Input: part model. Units: mm. Frame: model coordinates. Face numbers are marked on the shaded views. A direction names the side the tool comes from. Round coordinates to 2 decimals unless told otherwise and drop trailing zeros. Loops run counter-clockwise (first coordinate to the right, second up) from the corner with the lowest first, then second, coordinate; pieces in that order, holes last. Notation, with made-up numbers: (-6, 37.25) -> (8, 37.25) arc R22 ccw to (8, 71.25) -> close; hole circle Ø4 at (-12, 42). An arc over 180 degrees is marked (long way). Answer as a JSON object with one key per item and string values.
```python
from build123d import *

# Parameters (mm, degrees)
SKETCH_W        = 54.3
SKETCH_H        = 38
PAD_DEPTH       = 2
SKETCH001_W     = 54.3
SKETCH001_H     = 2
PAD001_DEPTH    = 22
SKETCH002_R     = 2.95
PAD002_DEPTH    = 5
SKETCH003_W     = 40
SKETCH003_H     = 22
PAD003_DEPTH    = 2
SKETCH004_W     = 40
SKETCH004_H     = 22
PAD004_DEPTH    = 2
SKETCH005_W     = 6.85
SKETCH005_H     = 15
PAD005_DEPTH    = 8
SKETCH006_R     = 1.4
POCKET_DEPTH    = 15
FILLET_R        = 3
FILLET001_R     = 2
SKETCH007_W     = 6.85
SKETCH007_H     = 25.8
PAD006_DEPTH    = 20
SKETCH008_R     = 1.4
POCKET001_DEPTH = 15
PAD007_DEPTH    = 2
SKETCH010_R     = 1.4
PAD008_DEPTH    = 2
SKETCH011_R     = 1.4
PAD009_DEPTH    = 2


with BuildPart() as body:
    # Sketch → Pad (new body)
    with BuildSketch(Plane.XY):
        with Locations((27.15, 21)):
            Rectangle(SKETCH_W, SKETCH_H)
    extrude(amount=PAD_DEPTH)

    # Sketch001 → Pad001 (join)
    with BuildSketch(Plane.XY):
        with Locations((27.15, 1)):
            Rectangle(SKETCH001_W, SKETCH001_H)
    extrude(amount=PAD001_DEPTH)

    # Sketch002 → Pad002 (join)
    with BuildSketch(Plane.XZ):
        with Locations((37.25, 12)):
            Circle(SKETCH002_R)
    extrude(amount=PAD002_DEPTH)

    # Sketch003 (on Face2 of Pad002) → Pad003 (join)
    with BuildSketch(Plane(origin=(0, 0, 0), x_dir=(0, -1, 0), z_dir=(-1, 0, 0))):
        with Locations((-20, 11)):
            Rectangle(SKETCH003_W, SKETCH003_H)
    extrude(amount=PAD003_DEPTH)

    # Sketch004 (on Face3 of Pad003) → Pad004 (join)
    with BuildSketch(Plane.YZ.offset(54.3)):
        with Locations((20, 11)):
            Rectangle(SKETCH004_W, SKETCH004_H)
    extrude(amount=PAD004_DEPTH)

    # Sketch005 (on Face5 of Pad004) → Pad005 (join)
    with BuildSketch(Plane.XY.offset(2)):
        with Locations((50.875, 20.3)):
            Rectangle(SKETCH005_W, SKETCH005_H)
    extrude(amount=PAD005_DEPTH)

    # Sketch006 (on Face15 of Pad005) → Pocket (cut)
    with BuildSketch(Plane(origin=(0, 27.8, 0), x_dir=(-1, 0, 0), z_dir=(0, 1, 0))):
        with Locations((-51.3, 7)):
            Circle(SKETCH006_R)
    extrude(amount=-POCKET_DEPTH, mode=Mode.SUBTRACT)

    # Fillet
    fillet_edges = [body.edges().sort_by_distance(p)[0] for p in [
        (47.45, 20.3, 10),
    ]]
    fillet(fillet_edges, radius=FILLET_R)

    # Fillet001
    fillet001_edges = [body.edges().sort_by_distance(p)[0] for p in [
        (52.375, 12.8, 10),
    ]]
    fillet(fillet001_edges, radius=FILLET001_R)

    # Sketch007 (on Face5 of Fillet001) → Pad006 (join)
    with BuildSketch(Plane.XY.offset(2)):
        with Locations((3.425, 14.9)):
            Rectangle(SKETCH007_W, SKETCH007_H)
    extrude(amount=PAD006_DEPTH)

    # Sketch008 (on Face14 of Pad006) → Pocket001 (cut)
    with BuildSketch(Plane(origin=(0, 27.8, 0), x_dir=(-1, 0, 0), z_dir=(0, 1, 0))):
        with Locations((-3, 7)):
            Circle(SKETCH008_R)
        with Locations((-3, 17)):
            Circle(SKETCH008_R)
    extrude(amount=-POCKET001_DEPTH, mode=Mode.SUBTRACT)

    # Sketch009 (on Face21 of Pocket001) → Pad007 (join)
    with BuildSketch(Plane.XY.offset(22)):
        Polygon((54.3, 2), (54.3, 40), (56.3, 40), (56.3, 0), (-2, 0), (-2, 40), (6.85, 40), (6.85, 2), align=None)
    extrude(amount=PAD007_DEPTH)

    # Sketch010 (on Face22 of Pad007) → Pad008 (join)
    with BuildSketch(Plane.YZ.offset(6.85)):
        with BuildLine():
            Line((2, 24), (38, 24))
            Line((38, 29), (38, 24))
            ThreePointArc((38, 29), (37.326745, 31.511013), (35.487593, 33.348396))
            Line((35.487593, 33.348396), (9.497223, 48.331729))
            ThreePointArc((9.497223, 48.331729), (4.498612, 48.329325), (2, 44))
            Line((2, 44), (2, 24))
        make_face()
        with Locations((7, 44)):
            Circle(SKETCH010_R, mode=Mode.SUBTRACT)
        with Locations((32.980762, 29)):
            Circle(SKETCH010_R, mode=Mode.SUBTRACT)
    extrude(amount=-PAD008_DEPTH)

    # Sketch011 (on Face20 of Pad008) → Pad009 (join)
    with BuildSketch(Plane(origin=(54.3, 0, 0), x_dir=(0, -1, 0), z_dir=(-1, 0, 0))):
        with BuildLine():
            Line((-38, 24), (-38, 29))
            ThreePointArc((-35.487593, 33.348396), (-37.326745, 31.511013), (-38, 29))
            Line((-35.487593, 33.348396), (-9.497223, 48.331729))
            ThreePointArc((-2, 44), (-4.498612, 48.329325), (-9.497223, 48.331729))
            Line((-2, 44), (-2, 24))
            Line((-2, 24), (-38, 24))
        make_face()
        with Locations((-7, 44)):
            Circle(SKETCH011_R, mode=Mode.SUBTRACT)
        with Locations((-32.980762, 29)):
            Circle(SKETCH011_R, mode=Mode.SUBTRACT)
    extrude(amount=-PAD009_DEPTH)


with BuildPart() as part_mirroring:
    # Part__Mirroring: instance of Body
    add(body.part.mirror(Plane(origin=(0, 0, 0), x_dir=(0, -1, 0), z_dir=(1, 0, 0))))


solid = part_mirroring.part
```
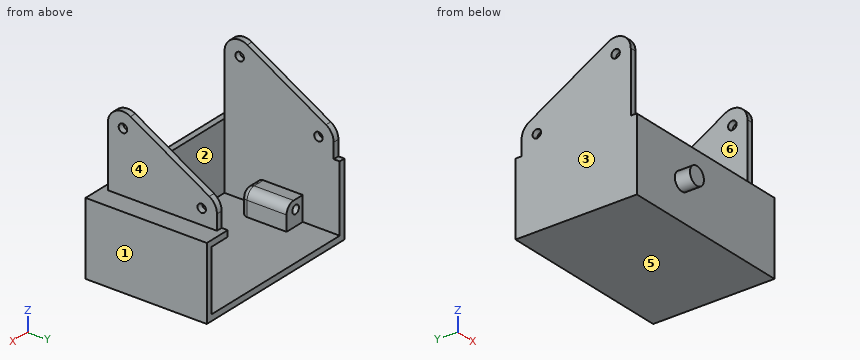
1) Draft query along X for the marked faces 1, 2 and 3. Return one class per face: +X half, -X half, draft (parallel to the pull), parting line (faces both ways), or undercut.
Output:
{"face 1": "+X half", "face 2": "undercut", "face 3": "-X half"}
2) Ray query, probe 1 along Z at (x, y) = (-3, 16); probe 2 along Z at (x, y) = (-1, 34.5); probe 3 along X at (y, z) = (12.5, 26). Return the intervals inside material, ascending.
Output:
{"probe 1": "z = 0 to 5.6, 8.4 to 15.6, 18.4 to 24", "probe 2": "z = 0 to 2, 22 to 24", "probe 3": "x = -56.3 to -54.3, -6.85 to -4.85"}
3) Section B-B, the plane y = 7. Output: boundary loops of the cut face in (x, z).
Output:
{"outline": "(-56.3, 0) -> (2, 0) -> (2, 24) -> (-4.85, 24) -> (-4.85, 42.6) -> (-6.85, 42.6) -> (-6.85, 2) -> (-54.3, 2) -> (-54.3, 42.6) -> (-56.3, 42.6) -> close; (-56.3, 45.4) -> (-54.3, 45.4) -> (-54.3, 49) -> (-56.3, 49) -> close; (-6.85, 45.4) -> (-4.85, 45.4) -> (-4.85, 49) -> (-6.85, 49) -> close"}
4) Section A-A, the plane z = 25. Output: boundary loops of the cut face in (x, y), plus the area to 3 significant figures.
Output:
{"outline": "(-56.3, 2) -> (-54.3, 2) -> (-54.3, 38) -> (-56.3, 38) -> close; (-6.85, 2) -> (-4.85, 2) -> (-4.85, 38) -> (-6.85, 38) -> close", "area": "144 mm^2"}
5) Section D-D, the plane y = 21.5. Output: boundary loops of the cut face in (x, z).
Output:
{"outline": "(-56.3, 0) -> (2, 0) -> (2, 24) -> (-4.85, 24) -> (-4.85, 41.41) -> (-6.85, 41.41) -> (-6.85, 2) -> (-47.45, 2) -> (-47.45, 7) arc R3 ccw to (-50.45, 10) -> (-54.3, 10) -> (-54.3, 41.41) -> (-56.3, 41.41) -> close; hole circle Ø2.8 at (-51.3, 7); hole circle Ø2.8 at (-3, 7); hole circle Ø2.8 at (-3, 17)"}
6) Section C-C, the plane x = -3. Output: boundary loops of the cut face in (y, z), plus the area to 3 significant figures.
Output:
{"outline": "(0, 0) -> (40, 0) -> (40, 2) -> (27.8, 2) -> (27.8, 5.6) -> (12.8, 5.6) -> (12.8, 8.4) -> (27.8, 8.4) -> (27.8, 15.6) -> (12.8, 15.6) -> (12.8, 18.4) -> (27.8, 18.4) -> (27.8, 22) -> (40, 22) -> (40, 24) -> (0, 24) -> close", "area": "632 mm^2"}
7) Reachability of the marked faces 4, 5 and 6 from +Z, -Z, +X, -X, +Y, -Y: full face, straight path, thin tool, end or side. Return the list, or none.
Output:
{"face 4": "+Z, +X, +Y, -Y", "face 5": "-Z, +X, -X, +Y, -Y", "face 6": "+Z, +Y"}
8) Contact query for flat-ended pins moving along their axis: P1, Ø1.6, axis at x = -6, z = 27, coming from the +Y side; P2, Ø12, axis at x = -23, y = 26, coming from the +Z side; P3, Ø5, axis at y = 0.5, z = 41, coming from the +X side; P4, Ø7.5, axis at x = -2.5, y = 31, coming from the -Z side. Output: stop coordinate, or through.
Output:
{"P1": "stops at y = 38", "P2": "stops at z = 2", "P3": "stops at x = -4.85", "P4": "stops at z = 0"}
